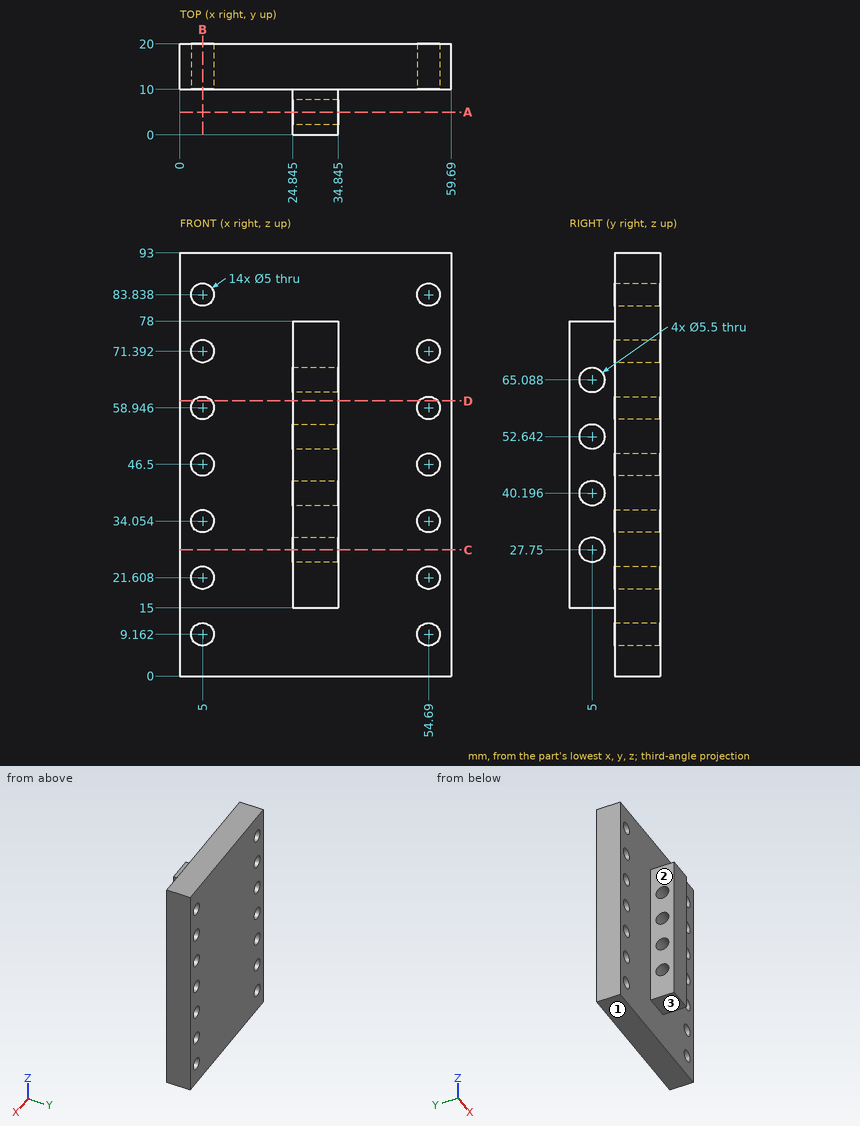
Geometry check sheet. Reference: drawing and pictorial views, mm from the part's lowest x, y, z. A direction names the side the tool comes from. Round coordinates to 2 decimals unless told otherwise and drop trailing zeros. Order: outer loops, then holes, each group sorted by start corner. A loop starts at its lowest first (then second) coordinate and runs counter-clockwise, first axis right, second up. Notation, with made-up numbers: M 84.25,-33 L 122.25,-33 A8 cw 122.25,-29 Z; hole C 81,-26 d4. An arc over 180 degrees is marked long. Answer in a Markdown table with one row per item.
(1) Sectioned sample at B-B, the plane x = 5. State how many separate pieces and enclosed holes the cut face has, and give its area (3 significant figures).
Responses:
| item | result |
|---|---|
| separate pieces | 8 |
| enclosed holes | 0 |
| area | 580 mm² |
(2) Sectioned sample at A-A, the plane y = 5. Record the cut outline in (x, z) (3 decimals).
Responses:
| item | result |
|---|---|
| outline | M 24.845,15 L 34.845,15 L 34.845,25 L 24.845,25 Z; M 24.845,30.5 L 34.845,30.5 L 34.845,37.446 L 24.845,37.446 Z; M 24.845,42.946 L 34.845,42.946 L 34.845,49.892 L 24.845,49.892 Z; M 24.845,55.392 L 34.845,55.392 L 34.845,62.338 L 24.845,62.338 Z; M 24.845,67.838 L 34.845,67.838 L 34.845,78 L 24.845,78 Z |
(3) Sectioned sample at C-C, the plane z = 27.75. Record the cut outline in (x, y) (3 decimals), and give its area (3 significant figures).
Responses:
| item | result |
|---|---|
| outline | M 0,10 L 24.845,10 L 24.845,7.75 L 34.845,7.75 L 34.845,10 L 59.69,10 L 59.69,20 L 0,20 Z; M 24.845,0 L 34.845,0 L 34.845,2.25 L 24.845,2.25 Z |
| area | 642 mm² |
(4) Scan lines: probe 1 along Z at (x, y) = (28, 5.25); probe 2 along Y at (x, z) = (46, 65); probe 3 along Z at (x, y) = (27, 1). Record each from-to range of solid material in increasing order. Write a range as from..to.
Responses:
| item | result |
|---|---|
| probe 1 | z = 15..25.01, 30.49..37.46, 42.93..49.9, 55.38..62.35, 67.83..78 |
| probe 2 | y = 10..20 |
| probe 3 | z = 15..78 |
(5) Tool access check on the marked faces 1, 2 and 3. Record the directions out of +Z, -Z, +X, -X, +Y, -Y that give a thin tool (end or side, any length) a straight path to the whole face; none if there is none.
Responses:
| item | result |
|---|---|
| face 1 | -Z, +X, -X, +Y, -Y |
| face 2 | +Z, -Z, -X, -Y |
| face 3 | -Z, +X, -X, -Y |
(6) Sectioned sample at D-D, the plane z = 60.5. Record the cut outline in (x, y) (3 decimals), and give its area (3 significant figures).
Responses:
| item | result |
|---|---|
| outline | M 0,10 L 3.042,10 L 3.042,20 L 0,20 Z; M 6.958,10 L 24.845,10 L 24.845,0 L 34.845,0 L 34.845,10 L 52.732,10 L 52.732,20 L 6.958,20 Z; M 56.648,10 L 59.69,10 L 59.69,20 L 56.648,20 Z |
| area | 619 mm² |
(7) Go/stop test with flat-tipped pins: P1, Ø3, axis at x = 27.5, y = 5.5, coming from the -Z side; P2, Ø9, axis at y = 5, z = 52.642, coming from the -X side (3 decimals); P3, Ø8, axis at x = 51, z = 26, coming from the -Y side. Record where each tip stops, or that it passes through.
Responses:
| item | result |
|---|---|
| P1 | stops at z = 15 |
| P2 | stops at x = 24.845 |
| P3 | stops at y = 10 |
